Verification items for the finished model (mm, model axes). A direction names the side the tool comes from. Give positions to 0.01 mm unless a question says otherwise; leave off trailing zeros. Order: outer loops, then holes, each group sorted by start corner. A loop starts at its lowest first (then second) coordinate and runs counter-clockwise, first axis right, second up. Notation, with made-up numbers: (-26, -39.5) - (-1, -39.5) arc R15 ccw to (-1, -24.5) - close; hole circle Ø6 at (66, 64.25). An arc over 180 degrees is marked (long way). Answer as a JSON object with one key per item and string values. Group by question number.
(1) Section check B-B (x = 5.5). Record the boundary of the cut face in (y, z).
(2) Thickness scan on line 1 (Y direction, x = 7, z = 2.5); line 2 (Z direction, x = -4, y = -71.5); line 3 (Y direction, x = -3.75, z = 6.5). Record the ranges inside material, lowest first.
(3) Section check C-C (y = -83). Record the boundary of the cut face in (x, z).
(4) Depth check by flat-ended pin: pin 1 Ø3 at (x, z) = (0.5, 15) entering from -Y; pin 2 Ø2 at (y, z) = (-85.5, 13.5) entering from +X; pin 3 Ø6 at (x, y) = (9.5, -66) entering from +Z. Enter the tip coordinate at first touch or a pass-through.
(5) Section check D-D (x = -5). Record the boundary of the cut face in (y, z), then the cut area to 3 significant figures.
(6) Section check A-A (z = 4). Record the boundary of the cut face in (x, y), then the cut area to 4 significant figures.
(7) Access from +Z, -Z, +X, -X, +Y, -Y to the whole of each face (thin tool, end or side, straight path). Record for faces 1 (the face through (9.539, -86, 13)), 2 (the face through (-2.336, -64, 4)), 3 (the face through (7.914, -64, 4)).
(8) Mould release check, pull along Y, two halves, no side actions. Record for faces 4 (the face through (-4.84, -69.21, 0.74)), 5 (the face through (3, -93.872, 6)), 6 (the face through (-6.211, -88, 6)): +Y half, -Y half, draft (parallel to the pull), parting line (faces both ways), or undercut.
```python
from build123d import *

# Parameters (mm, degrees)
EXTRUDE_1_DEPTH      = 1.5
SKETCH_2_W           = 18
SKETCH_2_H           = 12.5
EXTRUDE_2_DEPTH      = 9
SKETCH_3_W           = 13.5
SKETCH_3_H           = 2.47224136
EXTRUDE_3_DEPTH      = 6
SKETCH_4_W           = 10.25
SKETCH_4_H           = 6
EXTRUDE_4_DEPTH      = 5.6
HOLE_WIZARD_M2_5_1_D = 2.55


with BuildPart() as part:
    # 草圖1 → 填料-伸長1 (new body)
    with BuildSketch(Plane.XY):
        with BuildLine():
            Line((-6.760595539, -60.971994299), (12.339404461, -60.971994299))
            ThreePointArc((12.339404461, -60.971994299), (13.400064632, -61.411334127), (13.839404461, -62.471994299))
            Line((13.839404461, -62.471994299), (13.839404461, -93.871994299))
            ThreePointArc((13.839404461, -93.871994299), (13.400064632, -94.932654471), (12.339404461, -95.371994299))
            Line((12.339404461, -95.371994299), (-6.760595539, -95.371994299))
            ThreePointArc((-6.760595539, -95.371994299), (-7.821255711, -94.932654471), (-8.260595539, -93.871994299))
            Line((-8.260595539, -93.871994299), (-8.260595539, -62.471994299))
            ThreePointArc((-8.260595539, -62.471994299), (-7.821255711, -61.411334127), (-6.760595539, -60.971994299))
        make_face()
    extrude(amount=EXTRUDE_1_DEPTH)

    # 草圖2 → 填料-伸長2 (add)
    with BuildSketch(Plane.XY.offset(1.5)):
        with Locations((2.789404461, -87.621994299)):
            Rectangle(SKETCH_2_W, SKETCH_2_H)
    extrude(amount=EXTRUDE_2_DEPTH)

    # 草圖3 → 填料-伸長3 (add)
    with BuildSketch(Plane.XY.offset(10.5)):
        with Locations((2.789404461, -85.608114979)):
            Rectangle(SKETCH_3_W, SKETCH_3_H)
    extrude(amount=EXTRUDE_3_DEPTH)

    # 草圖4 → 填料-伸長4 (add)
    with BuildSketch(Plane.XY.offset(1.5)):
        with Locations((2.789404461, -63.971994299)):
            Rectangle(SKETCH_4_W, SKETCH_4_H)
    extrude(amount=EXTRUDE_4_DEPTH)

    # M2.5 螺旋的螺孔鑽1 (through all)
    with Locations(Plane.XY.offset(1.5)):
        with Locations((-5.010595539, -70.471994299), (10.589404461, -70.471994299)):
            Hole(HOLE_WIZARD_M2_5_1_D / 2)


solid = part.part
```
Solutions:
{
 "1": {"outline": "(-95.37, 0) - (-60.97, 0) - (-60.97, 7.1) - (-66.97, 7.1) - (-66.97, 1.5) - (-81.37, 1.5) - (-81.37, 10.5) - (-84.37, 10.5) - (-84.37, 16.5) - (-86.84, 16.5) - (-86.84, 10.5) - (-93.87, 10.5) - (-93.87, 1.5) - (-95.37, 1.5) - close"},
 "2": {"line 1": "y = -93.87 to -81.37, -66.97 to -60.97", "line 2": "z = 0 to 1.5", "line 3": "y = -93.87 to -81.37"},
 "3": {"outline": "(-8.26, 0) - (13.84, 0) - (13.84, 1.5) - (11.79, 1.5) - (11.79, 10.5) - (-6.21, 10.5) - (-6.21, 1.5) - (-8.26, 1.5) - close"},
 "4": {"pin 1": "stops at y = -86.84", "pin 2": "stops at x = 9.54", "pin 3": "stops at z = 7.1"},
 "5": {"outline": "(-95.37, 0) - (-71.75, 0) - (-71.75, 1.5) - (-81.37, 1.5) - (-81.37, 10.5) - (-93.87, 10.5) - (-93.87, 1.5) - (-95.37, 1.5) - close; (-69.2, 0) - (-60.97, 0) - (-60.97, 1.5) - (-69.2, 1.5) - close", "area": "160 mm2"},
 "6": {"outline": "(-6.21, -93.87) - (11.79, -93.87) - (11.79, -81.37) - (-6.21, -81.37) - close; (-2.34, -66.97) - (7.91, -66.97) - (7.91, -60.97) - (-2.34, -60.97) - close", "area": "286.5 mm2"},
 "7": {"face 1": "+Z, +X, +Y, -Y", "face 2": "+Z, -X, +Y", "face 3": "+Z, +X, +Y"},
 "8": {"face 4": "undercut", "face 5": "-Y half", "face 6": "draft"}
}
